```python
from build123d import *

# Parameters (mm, degrees)
F1_DEPTH = 25.4
F0_R     = 6.35
F2_DEPTH = 152.4
F0_W     = 152.4
F0_H     = 38.1
F3_DEPTH = 152.4


with BuildPart() as f1:
    # F0 (on Front) → F1 (new body)
    with BuildSketch(Plane.XZ):
        Polygon((127, 101.6), (152.4, 101.6), (152.4, 139.7), (0, 139.7), (0, 101.6), align=None)
        Polygon((-127, 101.6), (0, 101.6), (0, 139.7), (-152.4, 139.7), (-152.4, 101.6), align=None)
    extrude(amount=F1_DEPTH)



with BuildPart() as f1b:
    # F0 (on Front) → F1, piece 2 (new body)
    with BuildSketch(Plane.XZ):
        with BuildLine():
            ThreePointArc((139.7, 63.5), (132.2605122421, 81.4605122421), (114.3, 88.9))
            Line((114.3, 88.9), (-114.3, 88.9))
            ThreePointArc((-114.3, 88.9), (-132.2605122421, 81.4605122421), (-139.7, 63.5))
            Line((-139.7, 63.5), (-139.7, -63.5))
            ThreePointArc((-139.7, -63.5), (-132.2605122421, -81.4605122421), (-114.3, -88.9))
            Line((-114.3, -88.9), (114.3, -88.9))
            ThreePointArc((114.3, -88.9), (132.2605122421, -81.4605122421), (139.7, -63.5))
            Line((139.7, -63.5), (139.7, 63.5))
        make_face()
        Circle(F0_R, mode=Mode.SUBTRACT)
    extrude(amount=F1_DEPTH)


with BuildPart() as f1_1:
    add(f1.part)

    add(f1b.part)  # F2 merges F1b
    # F0 (on Front) → F2 (join)
    with BuildSketch(Plane.XZ):
        Polygon((127, 101.6), (152.4, 101.6), (152.4, 139.7), (0, 139.7), (0, 101.6), align=None)
        with BuildLine():
            ThreePointArc((152.4, 76.2), (144.9605122421, 94.1605122421), (127, 101.6))
            Line((127, 101.6), (0, 101.6))
            Line((0, 101.6), (-127, 101.6))
            ThreePointArc((-127, 101.6), (-144.9605122421, 94.1605122421), (-152.4, 76.2))
            Line((-152.4, 76.2), (-152.4, -76.2))
            ThreePointArc((-152.4, -76.2), (-144.9605122421, -94.1605122421), (-127, -101.6))
            Line((-127, -101.6), (127, -101.6))
            ThreePointArc((127, -101.6), (144.9605122421, -94.1605122421), (152.4, -76.2))
            Line((152.4, -76.2), (152.4, 76.2))
        make_face()
        with BuildLine():
            Line((-114.3, 88.9), (114.3, 88.9))
            ThreePointArc((114.3, 88.9), (132.2605122421, 81.4605122421), (139.7, 63.5))
            Line((139.7, 63.5), (139.7, -63.5))
            ThreePointArc((139.7, -63.5), (132.2605122421, -81.4605122421), (114.3, -88.9))
            Line((114.3, -88.9), (-114.3, -88.9))
            ThreePointArc((-114.3, -88.9), (-132.2605122421, -81.4605122421), (-139.7, -63.5))
            Line((-139.7, -63.5), (-139.7, 63.5))
            ThreePointArc((-139.7, 63.5), (-132.2605122421, 81.4605122421), (-114.3, 88.9))
        make_face(mode=Mode.SUBTRACT)
        Polygon((-127, 101.6), (0, 101.6), (0, 139.7), (-152.4, 139.7), (-152.4, 101.6), align=None)
    extrude(amount=F2_DEPTH)

    # F0 (on Front) → F3 (join)
    with BuildSketch(Plane.XZ):
        with BuildLine():
            ThreePointArc((152.4, 76.2), (144.9605122421, 94.1605122421), (127, 101.6))
            Line((127, 101.6), (0, 101.6))
            Line((0, 101.6), (-127, 101.6))
            ThreePointArc((-127, 101.6), (-144.9605122421, 94.1605122421), (-152.4, 76.2))
            Line((-152.4, 76.2), (-152.4, -76.2))
            ThreePointArc((-152.4, -76.2), (-144.9605122421, -94.1605122421), (-127, -101.6))
            Line((-127, -101.6), (127, -101.6))
            ThreePointArc((127, -101.6), (144.9605122421, -94.1605122421), (152.4, -76.2))
            Line((152.4, -76.2), (152.4, 76.2))
        make_face()
        with BuildLine():
            Line((-114.3, 88.9), (114.3, 88.9))
            ThreePointArc((114.3, 88.9), (132.2605122421, 81.4605122421), (139.7, 63.5))
            Line((139.7, 63.5), (139.7, -63.5))
            ThreePointArc((139.7, -63.5), (132.2605122421, -81.4605122421), (114.3, -88.9))
            Line((114.3, -88.9), (-114.3, -88.9))
            ThreePointArc((-114.3, -88.9), (-132.2605122421, -81.4605122421), (-139.7, -63.5))
            Line((-139.7, -63.5), (-139.7, 63.5))
            ThreePointArc((-139.7, 63.5), (-132.2605122421, 81.4605122421), (-114.3, 88.9))
        make_face(mode=Mode.SUBTRACT)
        with Locations((-76.2, 158.75)):
            Rectangle(F0_W, F0_H)
        with Locations((76.2, 158.75)):
            Rectangle(F0_W, F0_H)
    extrude(amount=F3_DEPTH)


solid = f1_1.part
```
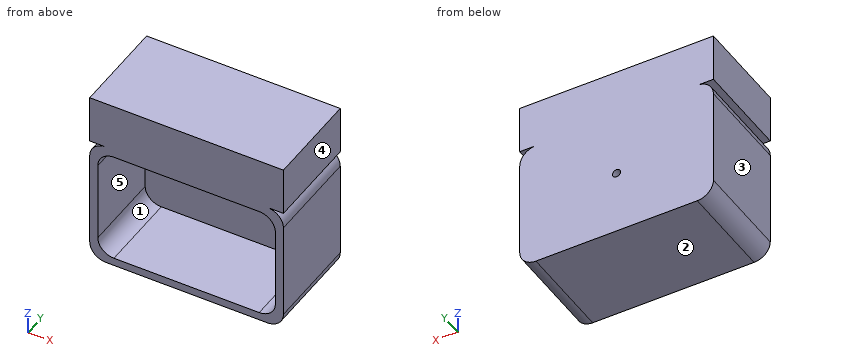
The listing builds one solid part. Answer for the finished solid, in the listing's coordinates (mm). Face numbers are marked on the shaded views. A direction names the side the tool comes from. Give positions to 0.01 mm unless a question says otherwise; leave off trailing zeros. Order: outer loops, then holes, each group sorted by start corner. A loop starts at its lowest first (then second) coordinate and runs counter-clockwise, first axis right, second up. Notation, with made-up numbers: M 28.25,-33.5 L 62.25,-33.5 A22 cw 62.25,-8.5 Z; hole C -35.5,29.5 d8. An arc over 180 degrees is marked long. Put each result on its own line as item: value. Start each with the question number.
Item 1: The part is cut by section A-A, the plane x = 0. Determine the outline of the cut face in (y, z).
Item 2: Flat-ended cylindrical pins translate along their axes: P1, Ø6, axis at y = -22, z = 87, coming from the -X side; P2, Ø7.5, axis at x = -142, y = -62, coming from the -Z side; P3, Ø3, axis at x = 31, z = -43.5, coming from the -Y side. Find the tip coordinate at first contact, or state that the pin passes through.
Item 3: The part is cut by section B-B, the plane z = 0. Determine the outline of the cut face in (x, y).
Item 4: The part is cut by section C-C, the plane y = -56. Determine the outline of the cut face in (x, z), and give its area (3 significant figures).
Item 5: Find the intervals of material crossed by line 1 along Z through (x, y) = (-41, -81.5); line 2 along Z through (x, y) = (0, -17); line 3 along X through (y, z) = (-55, -16), in increasing order.
Item 6: Which of the six approach directions +Z, -Z, +X, -X, +Y, -Y give full straight-line access (tool end or side, diameter ignored) to the marked faces 1 and 2?
Item 7: The part is cut by section D-D, the plane x = 105.5. Determine the outline of the cut face in (y, z), and give its area (3 significant figures).
Item 8: For a pull along X with two mould halves and no side action, classify the marked faces 3, 4 and 5 as +X half, -X half, draft (parallel to the pull), parting line (faces both ways), or undercut.
Answer key:
1. outline: M -152.4,-101.6 L 0,-101.6 L 0,-6.35 L -25.4,-6.35 L -25.4,-88.9 L -152.4,-88.9 Z; M -152.4,88.9 L -25.4,88.9 L -25.4,6.35 L 0,6.35 L 0,177.8 L -152.4,177.8 Z
2. P1: stops at x = -151.17
2. P2: stops at z = -98.97
2. P3: stops at y = -25.4
3. outline: M -152.4,-152.4 L -139.7,-152.4 L -139.7,-25.4 L -6.35,-25.4 L -6.35,0 L -152.4,0 Z; M 6.35,-25.4 L 139.7,-25.4 L 139.7,-152.4 L 152.4,-152.4 L 152.4,0 L 6.35,0 Z
4. outline: M -152.4,-76.2 A25.4 ccw -127,-101.6 L 127,-101.6 A25.4 ccw 152.4,-76.2 L 152.4,76.2 A25.4 ccw 127,101.6 L 152.4,101.6 L 152.4,177.8 L -152.4,177.8 L -152.4,101.6 L -127,101.6 A25.4 ccw -152.4,76.2 Z; hole M -139.7,-63.5 A25.4 ccw -114.3,-88.9 L 114.3,-88.9 A25.4 ccw 139.7,-63.5 L 139.7,63.5 A25.4 ccw 114.3,88.9 L -114.3,88.9 A25.4 ccw -139.7,63.5 Z
4. area: 35,500 mm²
5. line 1: z = -101.6 to -88.9, 88.9 to 177.8
5. line 2: z = -101.6 to -6.35, 6.35 to 177.8
5. line 3: x = -152.4 to -139.7, 139.7 to 152.4
6. face 1: -Y
6. face 2: -Z, +X, -X, +Y, -Y
7. outline: M -152.4,-101.6 L 0,-101.6 L 0,177.8 L -152.4,177.8 L -152.4,88.9 L -25.4,88.9 L -25.4,-88.9 L -152.4,-88.9 Z
7. area: 20,000 mm²
8. face 3: -X half
8. face 4: +X half
8. face 5: undercut
